Geometry check sheet. Reference: the model listing, model coordinates, mm. A direction names the side the tool comes from. Coordinates: 2 decimals unless noted, no trailing zeros. Loops run counter-clockwise (first coordinate to the right, second up) from the corner with the lowest first, then second, coordinate; pieces in that order, holes last.
from build123d import *

# Parameters (mm, degrees)
ESQUISSE1_W             = 122.76
ESQUISSE1_H             = 20
BOSS_EXTRU_1_DEPTH      = 6
ESQUISSE2_W             = 20
ESQUISSE2_H             = 6
BOSS_EXTRU_2_DEPTH      = 6
ESQUISSE3_R             = 1.5
ENL_V_MAT_EXTRU_1_DEPTH = 6


with BuildPart() as part:
    # Esquisse1 → Boss.-Extru.1 (new body)
    with BuildSketch(Plane.XY):
        Rectangle(ESQUISSE1_W, ESQUISSE1_H)
    extrude(amount=BOSS_EXTRU_1_DEPTH)

    # Esquisse2 → Boss.-Extru.2 (add)
    with BuildSketch(Plane.XY.offset(6)):
        with Locations((-36.38, -13)):
            Rectangle(ESQUISSE2_W, ESQUISSE2_H)
        with Locations((36.38, -13)):
            Rectangle(ESQUISSE2_W, ESQUISSE2_H)
    extrude(amount=-BOSS_EXTRU_2_DEPTH)

    # Esquisse3 → Enlèv. mat.-Extru.1 (cut)
    with BuildSketch(Plane.XY.offset(6)):
        with Locations((-36.38, -13)):
            Circle(ESQUISSE3_R)
        with Locations((36.38, -13)):
            Circle(ESQUISSE3_R)
    extrude(amount=-ENL_V_MAT_EXTRU_1_DEPTH, mode=Mode.SUBTRACT)


solid = part.part
(1) Sectioned sample at A-A on x = 36.38. Record the cut outline in (y, z).
Findings:
outline: (-16, 0) - (-14.5, 0) - (-14.5, 6) - (-16, 6) - close; (-11.5, 0) - (10, 0) - (10, 6) - (-11.5, 6) - close
(2) Scan lines: L1, parallel to Y at x = 36.38, z = 2.05; L2, parallel to X at y = -12.5, z = 2.6; L3, parallel to Y at x = 6, z = 1.6. Record each from-to range of solid material in increasing order.
Findings:
L1: y = -16 to -14.5, -11.5 to 10
L2: x = -46.38 to -37.79, -34.97 to -26.38, 26.38 to 34.97, 37.79 to 46.38
L3: y = -10 to 10
(3) Sectioned sample at B-B on y = -13. Record the cut outline in (x, z).
Findings:
outline: (-46.38, 0) - (-37.88, 0) - (-37.88, 6) - (-46.38, 6) - close; (-34.88, 0) - (-26.38, 0) - (-26.38, 6) - (-34.88, 6) - close; (26.38, 0) - (34.88, 0) - (34.88, 6) - (26.38, 6) - close; (37.88, 0) - (46.38, 0) - (46.38, 6) - (37.88, 6) - close
(4) Access from +Z, -Z, +X, -X, +Y, -Y to the whole of each face (thin tool, end or side, straight path). Record for faces 1 (the flat face through (36, -16, 3)), 2 (the flat face through (46.38, -13, 3)), 3 (the flat face through (-61.38, 0, 3)), 4 (the flat face through (-46.38, -13, 3)), 5 (the flat face through (-26.38, -13, 3)).
Findings:
face 1: +Z, -Z, +X, -X, -Y
face 2: +Z, -Z, +X, -Y
face 3: +Z, -Z, -X, +Y, -Y
face 4: +Z, -Z, -X, -Y
face 5: +Z, -Z, -Y
(5) Sectioned sample at D-D on x = 20.5. Record the cut outline in (y, z).
Findings:
outline: (-10, 0) - (10, 0) - (10, 6) - (-10, 6) - close
(6) Draft check along Y on faces 6 (the cylindrical face through (37.81, -12.55, 3.04)), 7 (the flat face through (-1, 10, 3)), 8 (the cylindrical face through (-37.88, -12.93, 3.04)), 9 (the flat face through (-1, -3, 6)). Enter one of: +Y half, -Y half, draft (parallel to the pull), parting line (faces both ways), or undercut.
Findings:
face 6: undercut
face 7: +Y half
face 8: undercut
face 9: draft
(7) Sectioned sample at C-C on z = 4.9. Record the cut outline in (x, y), and give its area (3 significant figures).
Findings:
outline: (-61.38, -10) - (-46.38, -10) - (-46.38, -16) - (-26.38, -16) - (-26.38, -10) - (26.38, -10) - (26.38, -16) - (46.38, -16) - (46.38, -10) - (61.38, -10) - (61.38, 10) - (-61.38, 10) - close; hole circle Ø3 at (-36.38, -13); hole circle Ø3 at (36.38, -13)
area: 2,680 mm2
(8) Gauge pin test, flat ends, axial feed: pin 1 Ø1.8 at (x, z) = (53.5, 4) entering from -Y; pin 2 Ø1.8 at (y, z) = (-14.5, 4) entering from +X; pin 3 Ø3 at (y, z) = (-13.5, 1.5) entering from -X. Record the tip position at first contact, or that the pin passes through.
Findings:
pin 1: stops at y = -10
pin 2: stops at x = 46.38
pin 3: stops at x = -46.38
